```python
from build123d import *

# Parameters (mm, degrees)
SALIENTE_EXTRUIR1_DEPTH      = 2.5
SALIENTE_EXTRUIR2_DEPTH      = 19
SALIENTE_EXTRUIR2_DEPTH_BACK = 19
CROQUIS3_R                   = 1
CORTAR_EXTRUIR2_DEPTH        = 2.5
CROQUIS2_W                   = 13
CROQUIS2_H                   = 5
CORTAR_EXTRUIR1_DEPTH        = 3
REDONDEO1_R                  = 1
CROQUIS7_W                   = 28
CROQUIS7_H                   = 15.287444166
CORTAR_EXTRUIR3_DEPTH        = 2.5
CROQUIS8_W                   = 5
CROQUIS8_H                   = 3
CORTAR_EXTRUIR4_DEPTH        = 2.5
REDONDEO2_R                  = 1
CROQUIS9_W                   = 5
CROQUIS9_H                   = 3
SALIENTE_EXTRUIR3_DEPTH      = 4.5
CROQUIS10_W                  = 5
CROQUIS10_H                  = 2
SALIENTE_EXTRUIR4_DEPTH      = 4
REDONDEO3_R                  = 1
REDONDEO3_OF_SIMETR_A3_R     = 1
REDONDEO4_R                  = 1


with BuildPart() as part:
    # Croquis1 → Saliente-Extruir1 (new body)
    with BuildSketch(Plane.XY):
        Polygon((-9, -15), (-14, -15), (-14, 15), (14, 15), (14, -15), (9, -15), (9, 5), (-9, 5), align=None)
    extrude(amount=SALIENTE_EXTRUIR1_DEPTH)

    # Croquis6 → Saliente-Extruir2 (add, two sides)
    with BuildSketch(Plane(origin=(0, 0, 0), x_dir=(0, 0, -1), z_dir=(1, 0, 0))) as saliente_extruir2_sk:
        Polygon((0, 14.99808723), (0, 11.497275395), (-11.558640634, 27.693398632), (-11.558640634, 31.194210467), align=None)
    extrude(amount=SALIENTE_EXTRUIR2_DEPTH)
    extrude(saliente_extruir2_sk.sketch, amount=-SALIENTE_EXTRUIR2_DEPTH_BACK)

    # Croquis3 → Cortar-Extruir2 (cut)
    with BuildSketch(Plane.XY.offset(2.5)):
        with Locations((-11.75, -13)):
            Circle(CROQUIS3_R)
        with Locations((-11.75, 11)):
            Circle(CROQUIS3_R)
        with Locations((12, -13)):
            Circle(CROQUIS3_R)
        with Locations((12, 11)):
            Circle(CROQUIS3_R)
    extrude(amount=-CORTAR_EXTRUIR2_DEPTH, mode=Mode.SUBTRACT)

    # Croquis2 → Cortar-Extruir1 (cut)
    with BuildSketch(Plane.XY.offset(2.5)):
        with Locations((0, 11.5)):
            Rectangle(CROQUIS2_W, CROQUIS2_H)
    extrude(amount=-CORTAR_EXTRUIR1_DEPTH, mode=Mode.SUBTRACT)

    # Redondeo1
    redondeo1_edges = [part.edges().sort_by_distance(p)[0] for p in [
        (14, -15, 1.25),
        (9, -15, 1.25),
        (9, 5, 1.25),
        (-9, 5, 1.25),
        (-9, -15, 1.25),
        (-14, -15, 1.25),
        (-6.5, 9, 1.25),
        (-6.5, 14, 1.25),
        (6.5, 14, 1.25),
        (6.5, 9, 1.25),
    ]]
    fillet(redondeo1_edges, radius=REDONDEO1_R)

    # Croquis7 → Cortar-Extruir3 (cut)
    with BuildSketch(Plane(origin=(0, 5.061109194, -7.091694501), x_dir=(-1, 0, 0), z_dir=(0, 0.580904735, -0.813971553))):
        with Locations((0, 24.46194693)):
            Rectangle(CROQUIS7_W, CROQUIS7_H)
    extrude(amount=-CORTAR_EXTRUIR3_DEPTH, mode=Mode.SUBTRACT)

    # Croquis8 → Cortar-Extruir4 (cut)
    with BuildSketch(Plane(origin=(0, 5.061109194, -7.091694501), x_dir=(-1, 0, 0), z_dir=(0, 0.580904735, -0.813971553))):
        with Locations((-16.5, 30.605669013)):
            Rectangle(CROQUIS8_W, CROQUIS8_H)
    cortar_extruir4 = extrude(amount=-CORTAR_EXTRUIR4_DEPTH, mode=Mode.SUBTRACT)

    # Simetría1: Cortar-Extruir4 across plane
    add(cortar_extruir4.mirror(Plane(origin=(0, 0, 0), x_dir=(0, 0, 1), z_dir=(1, 0, 0))), mode=Mode.SUBTRACT)

    # Redondeo2
    redondeo2_edges = [part.edges().sort_by_distance(p)[0] for p in [
        (16.5, 28.752295807, 9.815926431),
        (-16.5, 28.752295807, 9.815926431),
    ]]
    fillet(redondeo2_edges, radius=REDONDEO2_R)

    # Croquis9 → Saliente-Extruir3 (add)
    with BuildSketch(Plane(origin=(0, 3.879759153, -5.436370882), x_dir=(1, 0, 0), z_dir=(0, -0.580904735, 0.813971553))):
        with Locations((-16.5, 23.605669013)):
            Rectangle(CROQUIS9_W, CROQUIS9_H)
    saliente_extruir3 = extrude(amount=SALIENTE_EXTRUIR3_DEPTH)

    # Croquis10 → Saliente-Extruir4 (add)
    with BuildSketch(Plane(origin=(0, 20.4353004, 14.584001994), x_dir=(1, 0, 0), z_dir=(0, 0.813971553, 0.580904735))):
        with Locations((-16.5, 3.178821712)):
            Rectangle(CROQUIS10_W, CROQUIS10_H)
    saliente_extruir4 = extrude(amount=SALIENTE_EXTRUIR4_DEPTH)

    # Redondeo3
    redondeo3_edges = [part.edges().sort_by_distance(p)[0] for p in [
        (-16.5, 21.873144894, 7.404916908),
        (-16.5, 19.259073588, 11.067788897),
        (-16.5, 24.956874461, 15.134122039),
    ]]
    fillet(redondeo3_edges, radius=REDONDEO3_R)

    # Simetría3: Saliente-Extruir3, Saliente-Extruir4 across plane
    add(saliente_extruir3.mirror(Plane(origin=(0, 0, 0), x_dir=(0, 0, 1), z_dir=(1, 0, 0))))
    add(saliente_extruir4.mirror(Plane(origin=(0, 0, 0), x_dir=(0, 0, 1), z_dir=(1, 0, 0))))

    # Redondeo3 of Simetría3
    redondeo3_of_simetr_a3_edges = [part.edges().sort_by_distance(p)[0] for p in [
        (16.5, 21.873144894, 7.404916908),
        (16.5, 19.259073588, 11.067788897),
        (16.5, 24.956874461, 15.134122039),
    ]]
    fillet(redondeo3_of_simetr_a3_edges, radius=REDONDEO3_OF_SIMETR_A3_R)

    # Redondeo4
    redondeo4_edges = [part.edges().sort_by_distance(p)[0] for p in [
        (14, 18.159990774, 3.505753749),
        (-14, 18.159990774, 3.505753749),
    ]]
    fillet(redondeo4_edges, radius=REDONDEO4_R)


solid = part.part
```
Could you check a few things on this model? Use its own coordinates, in mm. A direction names the side the tool comes from. Coordinates: 2 decimals unless noted, no trailing zeros. Write each loop counter-clockwise with the first axis right and the second up, starting at its lowest first coordinate (ties: lowest second). Pieces come first, ordered by that corner, then holes. Notation, with made-up numbers: (72.5, 70.25) -> (96.5, 70.25) arc R18 ccw to (96.5, 76.25) -> close; hole circle Ø8 at (61, 33). An arc over 180 degrees is marked (long way). Return JSON: item names as keys, results as strings.
(1) Imagine slicing it at D-D, the plane z = 6.25. Please give me the cut outline in (x, y), then the cut area to 3 significant figures.
Numbers:
{"outline": "(-19, 20.25) -> (-14, 20.25) -> (-14, 23.76) -> (-19, 23.76) -> close; (14, 20.25) -> (19, 20.25) -> (19, 23.76) -> (14, 23.76) -> close", "area": "35.0 mm2"}
(2) Which directions (+Z, -Z, +X, -X, +Y, -Y) give clear straight access to the entire face, cutting with the end or side of a thin tool? Please do faces 1 (the flat face through (0, 7, 2.5)), 2 (the cylindrical face through (11.2, 10.4, 1.3)), 3 (the flat face through (-16.54, 20.58, 9.22)), 4 (the flat face through (0, 5, 1)), 5 (the flat face through (-16.54, 23.6, 10.15)).
Numbers:
{"face 1": "+Z, +X, -X, -Y", "face 2": "+Z, -Z", "face 3": "+X, -X, -Y", "face 4": "+Z, -Z, -Y", "face 5": "+X, -X"}
(3) Imagine slicing it at A-A, the plane x = 12. Count the separate pieces of the cut face and the enclosed holes in it, then the cut area to 3 significant figures.
Numbers:
{"separate pieces": "3", "enclosed holes": "0", "area": "72.9 mm2"}
(4) Imagine slicing it at B-B, the plane y = 11. Please give me the cut outline in (x, z).
Numbers:
{"outline": "(-14, 0) -> (-12.75, 0) -> (-12.75, 2.5) -> (-14, 2.5) -> close; (-10.75, 0) -> (-6.5, 0) -> (-6.5, 2.5) -> (-10.75, 2.5) -> close; (6.5, 0) -> (11, 0) -> (11, 2.5) -> (6.5, 2.5) -> close; (13, 0) -> (14, 0) -> (14, 2.5) -> (13, 2.5) -> close"}
(5) I'm going to push flat-ended pins straight in: pin 1 (3 mm diameter, centred on x = -0.5, z = 2, fed in from -Y); pin 2 (1.2 mm diameter, centred on x = -1, z = 1, fed in from +Y); pin 3 (1.2 mm diameter, centred on y = -3.5, z = 1.5, fed in from +X). Where does each tip first touch, or does it pass through?
Numbers:
{"pin 1": "stops at y = 5", "pin 2": "stops at y = 17.24", "pin 3": "stops at x = 14"}
(6) We'd pull the mould along Y, two halves only. Please class faces 6 (the flat face through (16.465, 25.92, 10.293)), 7 (the cylindrical face through (16.46, 28.34, 9.87)), 8 (the flat face through (-9, -5, 1)), 9 (the flat face through (-16.535, 25.92, 10.293)): +Y half, -Y half, draft (parallel to the pull), parting line (faces both ways), or undercut.
Numbers:
{"face 6": "undercut", "face 7": "+Y half", "face 8": "draft", "face 9": "undercut"}
(7) I need wall thicknesses on L1, parallel to X at y = 3.5, z = 1; L2, parallel to Y at x = 12, z = 0.8; L3, parallel to Y at x = -11.75, z = 0.9. Which ranges of each line are inside material? Lowest first, please.
Numbers:
{"L1": "x = -14 to -9, 9 to 14", "L2": "y = -15 to -14, -12 to 10, 12 to 16.12", "L3": "y = -15 to -14, -12 to 10, 12 to 16.26"}
